The listing builds one solid part. Answer for the finished solid, in the listing's coordinates (mm). Face numbers are marked on the shaded views. A direction names the side the tool comes from. Round coordinates to 2 decimals unless told otherwise and drop trailing zeros. Loops run counter-clockwise (first coordinate to the right, second up) from the corner with the lowest first, then second, coordinate; pieces in that order, holes last. Notation, with made-up numbers: (33.25, 1.5) - (55.25, 1.5) arc R26 cw to (55.25, 32.5) - close; hole circle Ø4 at (88, 45.25). An arc over 180 degrees is marked (long way). Write item = value, one per line. Start each with the question number.
1) Straight lines are drawn through the part: line 1 along Z through (x, y) = (0, -1.75); line 2 along Z through (x, y) = (-0.05, -6.75); line 3 along Z through (x, y) = (1.15, -3.5). For each, find the intervals that lie inside material, in ascending order.
2) Section A-A, the plane x = 0 is taken. Determine the outline of the cut face in (y, z).
3) Given pin 1 Ø2 at (x, z) = (-1, -8) entering from +Y; pin 2 Ø1 at (x, y) = (1.5, -6) entering from -Z, each flat-ended and moving along its own axis, determine where each tip first touches the part or whether it passes through.
4) Section D-D, the plane z = -2.75 is taken. Determine the outline of the cut face in (x, y).
5) Section B-B, the plane z = 1.5 is taken. Determine the outline of the cut face in (x, y), and give its area (3 significant figures).
6) Section C-C, the plane y = -3 is taken. Determine the outline of the cut face in (x, z).
7) A tool of negligible diameter and unlimited length cuts with its end or side. For the marked faces 1 and 2, from which of +Z, -Z, +X, -X, +Y, -Y can it reach the whole face along a straight path? Write none if from no direction.
8) For a pull along X with two mould halves and no side action, classify the marked faces 3 and 4 as released by +X, released by -X, zero draft, split by the parting line, or undercut.
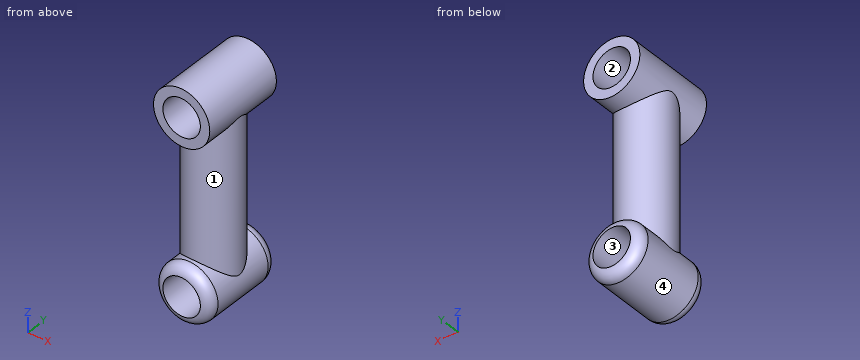
from build123d import *

# Parameters (mm, degrees)
F0_R     = 2.7
F0_R_2   = 1.8
F1_DEPTH = 8
F2_R     = 2.5
F3_DEPTH = 16
F4_DEPTH = 25
F5_R     = 2.7
F5_R_2   = 1.8
F6_DEPTH = 8
F7_DEPTH = 25


# Not quite as in the source:
# - a fillet or chamfer that OpenCascade refuses, or shapes differently, is made with other operations: its cross-section is extruded or revolved along the edge and cut away or added


with BuildPart() as f1:
    # F0 (on Front) → F1 (new body)
    with BuildSketch(Plane.XZ):
        with Locations((0, 0.773217123)):
            Circle(F0_R)
        with Locations((0, 0.773217123)):
            Circle(F0_R_2, mode=Mode.SUBTRACT)
    extrude(amount=F1_DEPTH)

    # F2 (on Top) → F3 (join)
    with BuildSketch(Plane.XY):
        with Locations((0, -4.1738846339)):
            Circle(F2_R)
    extrude(amount=-F3_DEPTH)

    # F0 (on Front) → F4 (cut)
    with BuildSketch(Plane.XZ):
        with Locations((0, 0.773217123)):
            Circle(F0_R_2)
    extrude(amount=F4_DEPTH, mode=Mode.SUBTRACT)

    # F5 (on Front) → F6 (join, through all)
    with BuildSketch(Plane.XZ):
        with Locations((0, -16.0034396241)):
            Circle(F5_R)
        with Locations((0, -16.0034396241)):
            Circle(F5_R_2, mode=Mode.SUBTRACT)
    extrude(amount=F6_DEPTH)

    # F5 (on Front) → F7 (cut)
    with BuildSketch(Plane.XZ):
        with Locations((0, -16.0034396241)):
            Circle(F5_R_2)
    extrude(amount=F7_DEPTH, mode=Mode.SUBTRACT)

    # F8: fillet of radius 1 on 1 edges, made by hand

    # F8_s1 → F8_t2 (revolve, cut)
    with BuildSketch(Plane.XY.offset(-16.0034396241)):
        with BuildLine():
            ThreePointArc((2.7, -0.9949874371), (2.4416198487, -0.3241670439), (1.8, 0))
            Line((1.8, 0), (2.7, 0))
            Line((2.7, 0), (2.7, -0.9949874371))
        make_face()
    revolve(axis=Axis((0, 0, -16.0034396241), (0, -1, 0)), mode=Mode.SUBTRACT)

    # F9: fillet of radius 1 on 1 edges, made by hand

    # F9_s1 → F9_t2 (revolve, cut)
    with BuildSketch(Plane.XY.offset(-16.0034396241)):
        with BuildLine():
            ThreePointArc((2.7, -7.0050125629), (2.4416198487, -7.6758329561), (1.8, -8))
            Line((1.8, -8), (2.7, -8))
            Line((2.7, -8), (2.7, -7.0050125629))
        make_face()
    revolve(axis=Axis((0, -8, -16.0034396241), (0, -1, 0)), mode=Mode.SUBTRACT)


solid = f1.part
Geometry check:
q1.line_1 = -18.7 to -17.8, -14.2 to -1.03, 2.57 to 3.47
q1.line_2 = -18.7 to -17.8, -14.2 to -13.3, -1.93 to -1.03, 2.57 to 3.47
q1.line_3 = -18.45 to -17.39, -14.62 to -0.61, 2.16 to 3.22
q2.outline = (-8, -17.8) arc R1 ccw to (-7.01, -18.7) - (-0.99, -18.7) arc R1 ccw to (0, -17.8) - close; (-8, -14.2) - (0, -14.2) arc R1 ccw to (-0.99, -13.3) - (-1.67, -13.3) - (-1.67, -1.93) - (0, -1.93) - (0, -1.03) - (-8, -1.03) - (-8, -1.93) - (-6.67, -1.93) - (-6.67, -13.3) - (-7.01, -13.3) arc R1 ccw to start; (-8, 2.57) - (0, 2.57) - (0, 3.47) - (-8, 3.47) - close
q3.pin_1 = -1.67
q3.pin_2 = -18.51
q4.outline = circle Ø5 at (0, -4.17)
q5.outline = (-2.6, -8) - (-1.65, -8) - (-1.65, 0) - (-2.6, 0) - close; (1.65, -8) - (2.6, -8) - (2.6, 0) - (1.65, 0) - close
q5.area = 15.3 mm2
q6.outline = (-2.21, -14.45) arc R2.7 ccw (long way) to (2.21, -14.45) - (2.21, -0.78) arc R2.7 ccw (long way) to (-2.21, -0.78) - close; hole circle Ø3.6 at (0, -16); hole circle Ø3.6 at (0, 0.77)
q7.face_1 = none
q7.face_2 = +Y, -Y
q8.face_3 = undercut
q8.face_4 = split by the parting line
